Could you check a few things on this model? Use its own coordinates, in mm. A direction names the side the tool comes from. Round coordinates to 2 decimals unless told otherwise and drop trailing zeros. Write each loop counter-clockwise with the first axis right and the second up, starting at its lowest first coordinate (ties: lowest second). Pieces come first, ordered by that corner, then holes. Notation, with made-up numbers: M -3.75,-27.75 L 0.25,-27.75 A27 ccw 0.25,3.25 Z; hole C 6.25,-27 d8. An arc over 180 degrees is marked long. One line per question, with ' | ' between items. Start each with the question number.
```python
from build123d import *

# Parameters (mm, degrees)
BOSS_EXTRUDE1_DEPTH = 60
SKETCH3_R           = 6
CUT_EXTRUDE1_DEPTH  = 24
CUT_EXTRUDE2_START  = -12
SKETCH3_3_R         = 6
CUT_EXTRUDE2_DEPTH  = 8
SKETCH4_R           = 2.75
CUT_EXTRUDE3_DEPTH  = 30


with BuildPart() as part:
    # Sketch1 → Boss-Extrude1 (new body)
    with BuildSketch(Plane.XY):
        Polygon((0, 0), (0, 60), (-26, 60), (-26, 20), (-56, 20), (-56, 0), (-16, 0), (-16, 50), (-10, 50), (-10, 0), align=None)
    extrude(amount=BOSS_EXTRUDE1_DEPTH)

    # Sketch3 → Cut-Extrude1 (cut)
    with BuildSketch(Plane(origin=(0, 20, 0), x_dir=(1, 0, 0), z_dir=(0, 1, 0))):
        with Locations(Location((-39.443747687, -30, 0), (0, 0, 180))):
            Circle(SKETCH3_R)
    extrude(amount=-CUT_EXTRUDE1_DEPTH, mode=Mode.SUBTRACT)

    # Sketch3<3> → Cut-Extrude2 (cut)
    with BuildSketch(Plane(origin=(0, 20, 0), x_dir=(1, 0, 0), z_dir=(0, 1, 0)).offset(CUT_EXTRUDE2_START)):
        Polygon((-31, -25.125), (-39.443747687, -20.25), (-47.887495374, -25.125), (-47.887495374, -34.875), (-39.443747687, -39.75), (-31, -34.875), align=None)
        with Locations(Location((-39.443747687, -30, 0), (0, 0, 180))):
            Circle(SKETCH3_3_R, mode=Mode.SUBTRACT)
    extrude(amount=-CUT_EXTRUDE2_DEPTH, mode=Mode.SUBTRACT)

    # Sketch4 → Cut-Extrude3 (cut)
    with BuildSketch(Plane.ZY.offset(26)):
        with Locations((14.458646622, 37.03116756)):
            Circle(SKETCH4_R)
        with Locations((45.541353378, 37.03116756)):
            Circle(SKETCH4_R)
    extrude(amount=-CUT_EXTRUDE3_DEPTH, mode=Mode.SUBTRACT)


solid = part.part
```
1. I'm going to push flat-ended pins straight in: P1, Ø5, axis at y = 37.03, z = 14.46, coming from the +X side; P2, Ø1, axis at y = 35, z = 23, coming from the +X side; P3, Ø3, axis at x = -13.5, z = 28.5, coming from the -Y side; P4, Ø14, axis at x = -39.44, z = 30, coming from the +Y side. Where does each tip first touch, or does it pass through?
2. Which directions (+Z, -Z, +X, -X, +Y, -Y) give clear straight access to the entire face, cutting with the end or side of a thin tool? Please do faces 5 (the face through (-35.2, 4.1, 22.7)), 6 (the face through (-5, 0, 30)), 7 (the face through (-26, 40, 30)), 8 (the face through (-21.07, 35.358, 12.276)), 9 (the face through (-13, 50, 30)).
3. Suppose I cut it at D-D (z = 47). Write out the boundary of the cut face in (x, y), and give its area (3 significant figures).
4. Suppose I cut it at B-B (y = 26.5). Write out the boundary of the cut face in (x, z).
5. I need wall thicknesses on line 1 along X through (y, z) = (31.5, 14); line 2 along X through (y, z) = (12.5, 7); line 3 along X through (y, z) = (51.5, 53). Which ranges of each line are inside material? Lowest first, please. Write a range as from..to.
6. If we mould it in two halves opening along X, with no side actions, what happens to faces 1 (the face through (-22, 24, 0)), 2 (the face through (-16, 25, 30)), 3 (the face through (0, 30, 30)), 4 (the face through (-42.212, 14.084, 24.677))? For each: released by +X, released by -X, zero draft, split by the parting line, or undercut.
7. Suppose I cut it at C-C (x = -36). Write out the boundary of the cut face in (y, z), and give its area (3 significant figures).
8. Suppose I cut it at A-A (z = 30). Write out the boundary of the cut face in (x, y), and give its area (3 significant figures).
Computed:
1) P1: passes through | P2: stops at x = 0 | P3: stops at y = 50 | P4: stops at y = 20
2) face 5: -Y | face 6: +Z, -Z, +X, -X, -Y | face 7: +Z, -Z, -X, +Y | face 8: +X, -X | face 9: +Z, -Z, -Y
3) outline: M -56,0 L -16,0 L -16,34.7 L -26,34.7 L -26,20 L -56,20 Z; M -26,39.36 L -16,39.36 L -16,50 L -10,50 L -10,39.36 L 0,39.36 L 0,60 L -26,60 Z; M -10,0 L 0,0 L 0,34.7 L -10,34.7 Z | area: 1,770 mm²
4) outline: M -26,0 L -16,0 L -16,60 L -26,60 Z; M -10,0 L 0,0 L 0,60 L -10,60 Z
5) line 1: x = -26..-16, -10..0 | line 2: x = -56..-16, -10..0 | line 3: x = -26..0
6) face 1: zero draft | face 2: undercut | face 3: released by +X | face 4: undercut
7) outline: M 0,0 L 20,0 L 20,25.09 L 8,25.09 L 8,22.24 L 0,22.24 Z; M 0,37.76 L 8,37.76 L 8,34.91 L 20,34.91 L 20,60 L 0,60 Z | area: 958 mm²
8) outline: M -56,0 L -47.89,0 L -47.89,8 L -45.44,8 L -45.44,20 L -56,20 Z; M -33.44,8 L -31,8 L -31,0 L -16,0 L -16,50 L -10,50 L -10,0 L 0,0 L 0,60 L -26,60 L -26,20 L -33.44,20 Z | area: 1,580 mm²
